Check sheet for the modelled part. Datum: model origin and axes. Units: mm. A direction names the side the tool comes from. Round coordinates to 2 decimals unless told otherwise and drop trailing zeros. Write each loop counter-clockwise with the first axis right and the second up, starting at its lowest first coordinate (ties: lowest second). Pieces come first, ordered by that corner, then holes.
Item 1: Section check D-D, the plane y = -18.5. Record the cut outline in (x, z).
Item 2: Section check A-A, the plane z = 3. Record the cut outline in (x, y), plus the area to 3 significant figures.
Item 3: Material ranges on line 1 along Y through (x, z) = (-27.4, 22.5); line 2 along X through (y, z) = (-32.5, 17); line 3 along Y through (x, z) = (-28.2, 22.5), recorded low to high.
Item 4: Depth check by flat-ended pin: pin 1 (6 mm diameter, centred on y = -29, z = 18, fed in from -X); pin 2 (1.5 mm diameter, centred on x = -27.5, z = 4.5, fed in from -Y); pin 3 (0.9 mm diameter, centred on x = -27.5, z = 5.5, fed in from +Y); pin 4 (2.5 mm diameter, centred on x = -7.5, y = 32.5, fed in from +Z). Enter the tip coordinate at first touch or a pass-through.
Item 5: Release check for a two-part mould opening along X. For faces 4 (the flat face through (-20, 25, 15)), 5 (the cylindrical face through (-6.801, 31.404, 15.036)), 6 (the cylindrical face through (-28.9, -24.43, 15.04)), 7 (the flat face through (-24, -24, 23)) record: pulls with the +X half, pulls with the -X half, needs draft (parallel to the pull), parting line crosses it, or undercut.
Item 6: Section check C-C, the plane z = 22.5. State how many separate pieces and enclosed holes the cut face has, plus the area to 3 significant figures.
Item 7: Section check B-B, the plane x = -18. Record the cut outline in (y, z), plus the area to 3 significant figures.
Item 8: Set-up check for faces 1 (the flat face through (-10.5, -30, 15)), 2 (the flat face through (-28, 10, 5)), 3 (the flat face through (-20, 22, 15)): record each of +Z, -Z, +X, -X, +Y, -Y from which the full face is reachable in a straight line by a thin tool's end or side.
Autodesk Inventor part; units mm, degrees
ref_plane "作業平面1" through (-29.5, -40, 30.5) normal (0, 0, -1) x (0, 1, 0)
ref_plane "YZ Plane" through (0, 0, 0) normal (1, 0, 0) x (0, 1, 0)
ref_plane "XZ Plane" through (0, 0, 0) normal (0, 1, 0) x (-1, 0, 0)
sketch "スケッチ1" plane through (0, 0, 0) normal (0, 0, 1) x (1, 0, 0)
  circle A0 centre (-7.5, -32.5) radius 1.6
  circle A1 centre (-7.5, 32.5) radius 1.6
  circle A2 centre (-7.5, -32.5) radius 1.3
  circle A3 centre (-7.5, 32.5) radius 1.3
  circle A4 centre (-7.5, 32.5) radius 3
  circle A5 centre (-7.5, -32.5) radius 3
  circle A6 centre (-7.5, 32.5) radius 1.6
  circle A7 centre (7.5, -32.5) radius 1.6
  circle A8 centre (7.5, 32.5) radius 1.6
  circle A9 centre (-7.5, -32.5) radius 1.6
  circle A10 centre (15.5, 0) radius 1.1
  circle A11 centre (10.5, -5) radius 1.1
  circle A12 centre (5.5, 0) radius 1.1
  circle A13 centre (10.5, 5) radius 1.1
  arc A14 (-10.5, -38) -> (-8.5, -40) centre (-8.5, -38) ccw
  line L0 (-8.5, -40) -> (8.5, -40)
  arc A15 (8.5, -40) -> (10.5, -38) centre (8.5, -38) ccw
  line L1 (10.5, -38) -> (10.5, -27)
  arc A16 (12.5, -25) -> (10.5, -27) centre (12.5, -27) ccw
  line L2 (12.5, -25) -> (18.5, -25)
  arc A17 (18.5, -25) -> (20.5, -23) centre (18.5, -23) ccw
  line L3 (20.5, -23) -> (20.5, 23)
  arc A18 (20.5, 23) -> (18.5, 25) centre (18.5, 23) ccw
  line L4 (18.5, 25) -> (12.5, 25)
  arc A19 (10.5, 27) -> (12.5, 25) centre (12.5, 27) ccw
  line L5 (10.5, 27) -> (10.5, 38)
  arc A20 (10.5, 38) -> (8.5, 40) centre (8.5, 38) ccw
  line L6 (8.5, 40) -> (-8.5, 40)
  arc A21 (-8.5, 40) -> (-10.5, 38) centre (-8.5, 38) ccw
  line L7 (-10.5, 38) -> (-10.5, 27)
  arc A22 (-12.5, 25) -> (-10.5, 27) centre (-12.5, 27) ccw
  line L8 (-12.5, 25) -> (-27.5, 25)
  arc A23 (-27.5, 25) -> (-29.5, 23) centre (-27.5, 23) ccw
  line L9 (-29.5, 23) -> (-29.5, -23)
  arc A24 (-29.5, -23) -> (-27.5, -25) centre (-27.5, -23) ccw
  line L10 (-27.5, -25) -> (-12.5, -25)
  arc A25 (-10.5, -27) -> (-12.5, -25) centre (-12.5, -27) ccw
  line L11 (-10.5, -27) -> (-10.5, -38)
  circle A26 centre (-8, 38) radius 1.1
  circle A27 centre (-8, -38) radius 1.1
  circle A28 centre (8, -38) radius 1.1
  circle A29 centre (8, 38) radius 1.1
  line L12 (-12.5, -22) -> (-26.5, -22)
  line L13 (-26.5, -22) -> (-26.5, 22)
  line L14 (-26.5, 22) -> (-12.5, 22)
  arc A30 (-12.5, 22) -> (-7.5, 27) centre (-12.5, 27) ccw
  line L15 (-7.5, 27) -> (-7.5, 37)
  line L16 (-7.5, 37) -> (7.5, 37)
  line L17 (7.5, 37) -> (7.5, 27)
  arc A31 (7.5, 27) -> (12.5, 22) centre (12.5, 27) ccw
  line L18 (12.5, 22) -> (17.5, 22)
  line L19 (17.5, 22) -> (17.5, -22)
  line L20 (17.5, -22) -> (12.5, -22)
  arc A32 (12.5, -22) -> (7.5, -27) centre (12.5, -27) ccw
  line L21 (7.5, -27) -> (7.5, -37)
  line L22 (7.5, -37) -> (-7.5, -37)
  line L23 (-7.5, -37) -> (-7.5, -27)
  arc A33 (-7.5, -27) -> (-12.5, -22) centre (-12.5, -27) ccw
  point P0 (0, 0)
  point P1 (-7.5, 29.5)
  point P2 (-10.5, 32.5)
  point P3 (-10.5, -32.5)
  point P4 (-7.5, -29.5)
  dimension "d0" = 2.6
  dimension "d1" = 2.6
  dimension "d2" = 6
  dimension "d3" = 6
  dimension "d4" = 3
ref_plane "作業平面1" through (-29.5, -40, 30.5) normal (0, 0, -1) x (0, 1, 0)
extrude "押し出し1" add sketch "スケッチ1" along normal up to surface (30.5 mm away) contours A0 L23 A2 | A0 L23 A5 | L23 A2 A0 | A0 L23 A5 | A5 L11 A25 L10 A24 L9 A23 L8 A22 L7 A4 L15 A30 L14 L13 L12 A33 L23 | L15 A1 A4 | A4 L15 A1 | L15 A3 A1 | A1 L15 A3
sketch "スケッチ2" plane through (-29.5, -23, 0) normal (-1, 0, 0) x (0, 0, 1)
  line L0 (0, 33) -> (10, 33)
  line L1 (10, 33) -> (10, 13)
  line L2 (10, 13) -> (0, 13)
  line L3 (0, 13) -> (0, 33)
  line L4 (0, 46) -> (0, 0)
  point P0 (0, 23)
  point P1 (10, 23)
  point P2 (0, 23)
  point P3 (0, 23)
  dimension "d7" = 10
  dimension "d8" = 20
extrude "押し出し2" cut sketch "スケッチ2" against normal through all
fillet "フィレット1" radius 2 4 edges at (-28, 10, 10) (-28, 10, 0) (-28, -10, 10) (-28, -10, 0)
sketch "スケッチ3" plane through (-27.5, -25, 0) normal (0, -1, 0) x (1, 0, 0)
  line L0 (15, 30.5) -> (1, 30.5)
  line L1 (3.5, 30.5) -> (12.5, 30.5)
  line L2 (12.5, 30.5) -> (12.5, 16.5)
  line L3 (12.5, 16.5) -> (3.5, 16.5)
  line L4 (3.5, 16.5) -> (3.5, 30.5)
  point P0 (27.5, 0)
  point P1 (8, 30.5)
  point P2 (8, 16.5)
  point P3 (12.5, 30.5)
  dimension "d12" = 9
  dimension "d13" = 14
extrude "押し出し3" cut sketch "スケッチ3" against normal up to surface (3 mm away)
sketch "スケッチ4" plane through (-29.5, -23, 30.5) normal (-1, 0, 0) x (0, 0, 1)
  circle A0 centre (-8, 41.5) radius 1.75
  circle A1 centre (-8, 4.5) radius 1.75
  line L0 (0, 46) -> (0, 0)
  point P0 (-30.5, 23)
  point P1 (0, 23)
  dimension "d16" = 3.5
  dimension "d17" = 3.5
  dimension "d18" = 37
  dimension "d19" = 18.5
  dimension "d20" = 8
extrude "押し出し4" cut sketch "スケッチ4" against normal through all
properties part number "mune_2" material "ABS プラスチック"
Values found:
1. outline: (-29.5, 0) - (-26.5, 0) - (-26.5, 20.75) - (-29.5, 20.75) - close; (-29.5, 24.25) - (-26.5, 24.25) - (-26.5, 30.5) - (-29.5, 30.5) - close
2. outline: (-29.5, -23) arc R2 ccw to (-27.5, -25) - (-12.5, -25) arc R2 cw to (-10.5, -27) - (-10.5, -32.5) arc R3 ccw (long way) to (-7.5, -29.5) - (-7.5, -27) arc R5 ccw to (-12.5, -22) - (-26.5, -22) - (-26.5, -10) - (-29.5, -10) - close; (-29.5, 10) - (-26.5, 10) - (-26.5, 22) - (-12.5, 22) arc R5 ccw to (-7.5, 27) - (-7.5, 29.5) arc R3 ccw (long way) to (-10.5, 32.5) - (-10.5, 27) arc R2 cw to (-12.5, 25) - (-27.5, 25) arc R2 ccw to (-29.5, 23) - close; hole circle Ø2.6 at (-7.5, -32.5); hole circle Ø2.6 at (-7.5, 32.5)
2. area: 270 mm2
3. line 1: y = -25 to -20.25, -16.75 to 16.75, 20.25 to 25
3. line 2: x = -10.5 to -8.8, -6.2 to -4.5
3. line 3: y = -24.87 to -20.25, -16.75 to 16.75, 20.25 to 24.87
4. pin 1: stops at x = -10.77
4. pin 2: stops at y = -25
4. pin 3: stops at y = 25
4. pin 4: passes through
5. face 4: needs draft
5. face 5: undercut
5. face 6: pulls with the -X half
5. face 7: undercut
6. separate pieces: 4
6. enclosed holes: 2
6. area: 282 mm2
7. outline: (-25, 0) - (-22, 0) - (-22, 16.5) - (-25, 16.5) - close; (22, 0) - (25, 0) - (25, 30.5) - (22, 30.5) - close
7. area: 141 mm2
8. face 1: +Z, -Z, -X, -Y
8. face 2: -Z, +X, -X
8. face 3: +Z, -Z, +X
